```python
from build123d import *

# Parameters (mm, degrees)
F0_W     = 31
F0_H     = 55
F1_DEPTH = 34
F2_T     = -2
F3_R     = 3
F4_DEPTH = 4


with BuildPart() as f1:
    # F0 (on Top) → F1 (new body)
    with BuildSketch(Plane.XY):
        Rectangle(F0_W, F0_H)
    extrude(amount=F1_DEPTH)

    # F2
    f2_openings = [f1.faces().sort_by_distance(p)[0] for p in [
        (15.5, 0, 17),
    ]]
    offset(amount=F2_T, openings=f2_openings)

    # F3 (on face) → F4 (cut)
    with BuildSketch(Plane(origin=(0, 0, 0), x_dir=(1, 0, 0), z_dir=(0, 0, -1))):
        with Locations((-11.5, -10.076838)):
            Circle(F3_R)
        with Locations((-11.5, 21.163162)):
            Circle(F3_R)
        with Locations((14.1, -10.076838)):
            Circle(F3_R)
        with Locations((14.1, 21.163162)):
            Circle(F3_R)
    extrude(amount=-F4_DEPTH, mode=Mode.SUBTRACT)


solid = f1.part
```
Source: CAD feature listing. Evaluate the final solid. Frame: model axes, mm. A direction names the side the tool comes from. Give positions to 0.01 mm unless a question says otherwise; leave off trailing zeros. Order: outer loops, then holes, each group sorted by start corner. A loop starts at its lowest first (then second) coordinate and runs counter-clockwise, first axis right, second up.
(1) Pull-direction query (Z, two-part tool) for faces 4 (the face through (0, 0, 34)), 5 (the face through (11.1, 10, 1)), 6 (the face through (1, 0, 2)); classes: +Z half, -Z half, draft (parallel to the pull), parting line (faces both ways), or undercut.
(2) Contact query for a flat-ended pin moving along its axis: P1, Ø0.5, axis at x = -14, y = 10, coming from the -Z side. Output: stop coordinate, or through.
(3) Section query B-B (y = -1.5). Return the cut outline in (x, z), plus the area to 3 significant figures.
(4) Access query for faces 1 (the face through (-14.497, 9.945, 1.528)), 2 (the face through (1, -25.5, 17)), 3 (the face through (0, -27.5, 17)). Directions: +Z, -Z, +X, -X, +Y, -Y. A direction counts if a zero-diameter tool reaches every point of the face in a straight line with its end or side. Return the directions, or none.
(5) Section query A-A (x = 14.1). Return the cut outline in (y, z), plus the area to 3 significant figures.
(6) Section query D-D (x = 5.5). Return the cut outline in (y, z).
(7) Material intervals for line 1 along Z through (x, y) = (3, 16.5); line 2 along Y through (x, z) = (8, 16); line 3 along X through (y, z) = (-4, 3.5), sorted ascending.
(8) Section query C-C (z = 29.5). Return the cut outline in (x, y).
Outcome:
1. face 4: +Z half
1. face 5: draft
1. face 6: undercut
2. P1: stops at z = 4
3. outline: (-15.5, 0) - (15.5, 0) - (15.5, 2) - (-13.5, 2) - (-13.5, 32) - (15.5, 32) - (15.5, 34) - (-15.5, 34) - close
3. area: 184 mm2
4. face 1: -Z
4. face 2: +X
4. face 3: +Z, -Z, +X, -X, -Y
5. outline: (-27.5, 0) - (-24.16, 0) - (-24.16, 2) - (-25.5, 2) - (-25.5, 32) - (25.5, 32) - (25.5, 2) - (13.08, 2) - (13.08, 0) - (27.5, 0) - (27.5, 34) - (-27.5, 34) - close; (-18.16, 0) - (7.08, 0) - (7.08, 2) - (-18.16, 2) - close
5. area: 316 mm2
6. outline: (-27.5, 0) - (27.5, 0) - (27.5, 34) - (-27.5, 34) - close; hole (-25.5, 2) - (25.5, 2) - (25.5, 32) - (-25.5, 32) - close
7. line 1: z = 0 to 2, 32 to 34
7. line 2: y = -27.5 to -25.5, 25.5 to 27.5
7. line 3: x = -15.5 to -13.5
8. outline: (-15.5, -27.5) - (15.5, -27.5) - (15.5, -25.5) - (-13.5, -25.5) - (-13.5, 25.5) - (15.5, 25.5) - (15.5, 27.5) - (-15.5, 27.5) - close
